```python
from build123d import *

# Parameters (mm, degrees)
SKETCH1_W           = 2
SKETCH1_H           = 2
BOSS_EXTRUDE1_DEPTH = 3
SKETCH2_R           = 0.5
CUT_EXTRUDE1_DEPTH  = 0.01
SKETCH3_R           = 0.35


with BuildPart() as part:
    # Sketch1 → Boss-Extrude1 (new body)
    with BuildSketch(Plane(origin=(0, 0, 0), x_dir=(1, 0, 0), z_dir=(0, 1, 0))):
        Rectangle(SKETCH1_W, SKETCH1_H)
    extrude(amount=BOSS_EXTRUDE1_DEPTH)

    # Sketch2 → Cut-Extrude1 (cut)
    with BuildSketch(Plane(origin=(0, 0, -1), x_dir=(-1, 0, 0), z_dir=(0, 0, -1))):
        with Locations((0.45, 1.500545884)):
            Circle(SKETCH2_R)
    extrude(amount=-CUT_EXTRUDE1_DEPTH, mode=Mode.SUBTRACT)

    # Sweep1: sweep along a path in Sketch8
    with BuildLine(Plane(origin=(-1, 1.5, 0), x_dir=(1, 0, 0), z_dir=(0, 0, 1))) as sweep1_path:
        Line((0, 0), (-0.152776169, 0))
        ThreePointArc((-0.152776169, 0), (-0.50632956, -0.146446609), (-0.652776169, -0.5))
        Line((-0.652776169, -0.5), (-0.652776169, -75.5))
    # Sketch3 → Sweep1 (sweep)
    with BuildSketch(Plane.ZY.offset(1)):
        with Locations((0, 1.5)):
            Circle(SKETCH3_R)
    sweep1 = sweep(path=sweep1_path.line)

    # Mirror1: Sweep1 across plane
    add(sweep1.mirror(Plane(origin=(0, 0, 0), x_dir=(0, 0, 1), z_dir=(1, 0, 0))))


solid = part.part
```
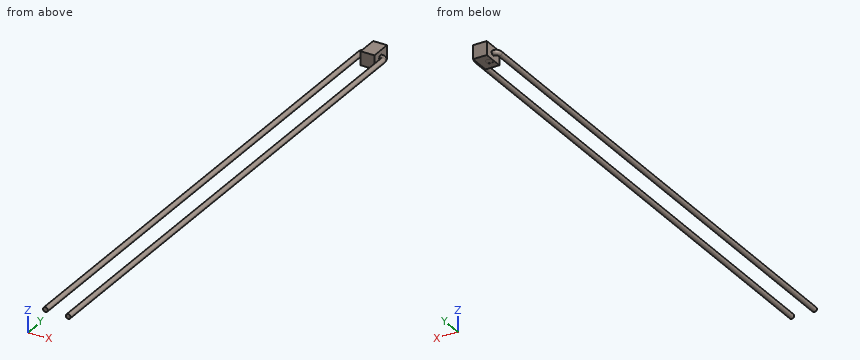
The model under review builds one solid part; all positions refer to its coordinate system, in mm. Round coordinates to 2 decimals unless told otherwise and drop trailing zeros. Order: outer loops, then holes, each group sorted by start corner. A loop starts at its lowest first (then second) coordinate and runs counter-clockwise, first axis right, second up. Notation, with made-up numbers: M 84,-26 L 113,-26 A23 ccw 113,10 Z; hole C 89.5,13.5 d9. An arc over 180 degrees is marked long. Use a Markdown table: item, result.
1) Insertion check: pin 1 (1 mm diameter, centred on x = 0, z = 0, fed in from -Y); pin 2 (0.8 mm diameter, centred on x = -0.5, y = 1.5, fed in from -Z). Each pin has a flat end and moves straight along its axis. Give the tip position at first contact, or say it passes through.
Report:
| item | result |
|---|---|
| pin 1 | y = 0 |
| pin 2 | z = -0.99 |
2) Wall thickness on line 1 along X through (y, z) = (-62, -0.05); line 2 along Y through (x, z) = (-0.45, -0.95); line 3 along X through (y, z) = (-9, 0.25): over which ranges is each line inside the solid? List them lowest first. Write a range as [from, to].
Report:
| item | result |
|---|---|
| line 1 | [-2, -1.31], [1.31, 2] |
| line 2 | [0, 3] |
| line 3 | [-1.9, -1.41], [1.41, 1.9] |
3) Consider section A-A (z = 0). Write out the cut boundary in (x, y), then the cut area to 3 significant figures.
Report:
| item | result |
|---|---|
| outline | M -2,-74 L -1.3,-74 L -1.3,1 A0.15 cw -1.15,1.15 L -1,1.15 L -1,0 L 1,0 L 1,1.15 L 1.15,1.15 A0.15 cw 1.3,1 L 1.3,-74 L 2,-74 L 2,1 A0.85 ccw 1.15,1.85 L 1,1.85 L 1,3 L -1,3 L -1,1.85 L -1.15,1.85 A0.85 ccw -2,1 Z |
| area | 112 mm^2 |
4) Consider section B-B (y = -60.5). Write out the cut boundary in (x, z), then the cut area to 3 significant figures.
Report:
| item | result |
|---|---|
| outline | C -1.65,0 d0.7; C 1.65,0 d0.7 |
| area | 0.770 mm^2 |
